Part print with two shaded views. Sizes in mm from the minimum x, y, z corner. A direction names the side the tool comes from. Give positions to 0.01 mm unless a question says otherwise; leave off trailing zeros. Order: outer loops, then holes, each group sorted by start corner. A loop starts at its lowest first (then second) coordinate and runs counter-clockwise, first axis right, second up. Notation, with made-up numbers: M 60,67.5 L 75,67.5 A25 ccw 75,106.5 Z; hole C 76.5,73 d8. An arc over 180 degrees is marked long. Return JSON: item names as keys, results as strings. Group by question number.
1. Slice it at D-D on x = 35.5. List the corners of the cut face in (y, z) (1 decimal), then the cut area to 3 significant figures.
2. Slice it at A-A on x = 5. List the corners of the cut face in (y, z) (1 decimal).
3. 3-axis set-ups, long thin cutter, end or side, ignore diameter. For the marked faces 5 and 6: which of +Z, -Z, +X, -X, +Y, -Y reach the whole face in a straight line?
4. Wall check: probe 1 along Z at (x, y) = (38.5, 30) (1 decimal); probe 2 along Y at (x, z) = (28.5, 27) (1 decimal); probe 3 along Y at (x, z) = (28, 24.5) (1 decimal). Give the ranges that are in metal, low to high. Write a range as [from, to].
5. Pin check, flat tips, straight feed: pin 1 (6 mm diameter, centred on x = 22, z = 50, fed in from +Y); pin 2 (9.5 mm diameter, centred on y = 35.75, z = 30.96, fed in from -X); pin 3 (10 mm diameter, centred on x = 21, y = 50, fed in from -Z); pin 4 (2 mm diameter, centred on x = 28, z = 42, fed in from -Y) (1 decimal). Stop position of each tip, or through.
6. Two-plate mould, pull along Y, no slides. Class the marked faces 1, 2, 3 and 4: released by +Y, released by -Y, zero draft, split by the parting line, or undercut.
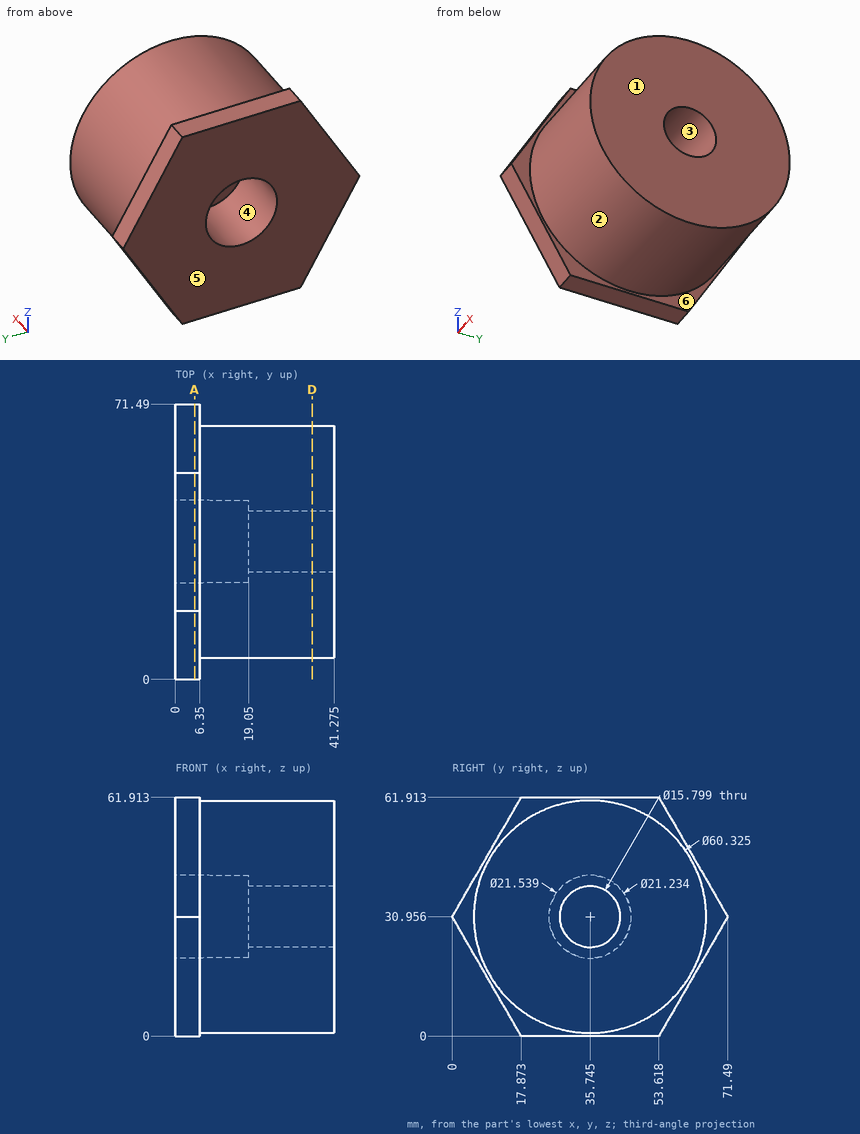
Result:
{
 "1": {"outline": "C 35.7,31 d60.3; hole C 35.7,31 d15.8", "area": "2,660 mm2"},
 "2": {"outline": "M 0,31 L 17.9,0 L 53.6,0 L 71.5,31 L 53.6,61.9 L 17.9,61.9 Z; hole C 35.7,31 d21.5"},
 "3": {"face 5": "+Z, -Z, -X, +Y, -Y", "face 6": "+X"},
 "4": {"probe 1": "z = [1.3, 25.5], [36.4, 60.6]", "probe 2": "y = [5.8, 28.9], [42.6, 65.6]", "probe 3": "y = [6.3, 31.2], [40.3, 65.2]"},
 "5": {"pin 1": "stops at y = 61.29", "pin 2": "passes through", "pin 3": "stops at z = 2.25", "pin 4": "stops at y = 7.3"},
 "6": {"face 1": "zero draft", "face 2": "split by the parting line", "face 3": "undercut", "face 4": "undercut"}
}
